from build123d import *

# Parameters (mm, degrees)
BOSS_EXTRUDE3_DEPTH              = 14.5
SKETCH8_R                        = 7.935
CUT_EXTRUDE3_DEPTH               = 88
CUT_EXTRUDE9_DEPTH               = 2.4
F_39_0_13779528_DIAMETER_HOLE1_D = 3.500000112
CUT_EXTRUDE10_DEPTH              = 22.4
CUT_EXTRUDE11_DEPTH              = 2.4
BOSS_EXTRUDE7_DEPTH              = 3.625
F_39_0_13779528_DIAMETER_HOLE2_D = 3.500000112
BOSS_EXTRUDE10_DEPTH             = 3
BOSS_EXTRUDE11_DEPTH             = 3


with BuildPart() as part:
    # Sketch6 → Boss-Extrude3 (new body)
    with BuildSketch(Plane(origin=(0, 0, 0), x_dir=(1, 0, 0), z_dir=(0, 1, 0))):
        Polygon((-16.836914056, 5.783353512), (13.163085944, 5.783353512), (20.663085944, -47.581919406), (-24.336914056, -47.581919406), align=None)
    extrude(amount=BOSS_EXTRUDE3_DEPTH)

    # Sketch8 → Cut-Extrude3 (cut)
    with BuildSketch(Plane.XY.offset(47.581919406)):
        with Locations((-1.836914056, 0)):
            Circle(SKETCH8_R)
    extrude(amount=-CUT_EXTRUDE3_DEPTH, mode=Mode.SUBTRACT)

    # Sketch18 → Cut-Extrude9 (cut)
    with BuildSketch(Plane(origin=(0, 14.5, 0), x_dir=(1, 0, 0), z_dir=(0, 1, 0))):
        Polygon((-15.771819769, -44.868285994), (-12.821819769, -43.1651027), (-12.821819769, -39.758736112), (-15.771819769, -38.055552818), (-18.721819769, -39.758736112), (-18.721819769, -43.1651027), align=None)
        Polygon((12.097991657, -44.868285994), (15.047991657, -43.1651027), (15.047991657, -39.758736112), (12.097991657, -38.055552818), (9.147991657, -39.758736112), (9.147991657, -43.1651027), align=None)
        Polygon((11.389331688, -26.016021021), (14.389331688, -24.283970214), (14.389331688, -20.819868599), (11.389331688, -19.087817791), (8.389331688, -20.819868599), (8.389331688, -24.283970214), align=None)
        Polygon((-15.0631598, -26.016021021), (-12.0631598, -24.283970214), (-12.0631598, -20.819868599), (-15.0631598, -19.087817791), (-18.0631598, -20.819868599), (-18.0631598, -24.283970214), align=None)
    extrude(amount=-CUT_EXTRUDE9_DEPTH, mode=Mode.SUBTRACT)

    # #39 (0.13779528) Diameter Hole1 (through all)
    with Locations(Plane(origin=(-15.0631598, 14.5, 22.551919406), x_dir=(0, 0, 1), z_dir=(0, 1, 0))):
        with Locations((0, 0), (0, 26.452491488), (18.91, -0.708659969), (18.91, 27.161151457)):
            Hole(F_39_0_13779528_DIAMETER_HOLE1_D / 2)

    # Sketch22 → Cut-Extrude10 (cut)
    with BuildSketch(Plane(origin=(0, 14.5, 0), x_dir=(1, 0, 0), z_dir=(0, 1, 0))):
        Polygon((-22.781301734, -36.51316259), (19.107473622, -36.51316259), (13.163085944, 5.783353512), (-16.836914056, 5.783353512), align=None)
    extrude(amount=-CUT_EXTRUDE10_DEPTH, mode=Mode.SUBTRACT)

    # Sketch24 → Cut-Extrude11 (cut)
    with BuildSketch(Plane.XZ):
        Polygon((-15.771819769, 38.055552818), (-12.821819769, 39.758736112), (-12.821819769, 43.1651027), (-15.771819769, 44.868285994), (-18.721819769, 43.1651027), (-18.721819769, 39.758736112), align=None)
        Polygon((12.097991657, 38.055552818), (15.047991657, 39.758736112), (15.047991657, 43.1651027), (12.097991657, 44.868285994), (9.147991657, 43.1651027), (9.147991657, 39.758736112), align=None)
    extrude(amount=-CUT_EXTRUDE11_DEPTH, mode=Mode.SUBTRACT)

    # Sketch27 → Boss-Extrude7 (add)
    with BuildSketch(Plane(origin=(0, 0, 0), x_dir=(1, 0, 0), z_dir=(0, 1, 0))):
        Polygon((6.098085944, -47.581919406), (20.663085944, -47.581919406), (20.663085944, -112.581919406), (-9.771914056, -112.581919406), (-24.336914056, -112.581919406), (-24.336914056, -47.581919406), (-9.771914056, -47.581919406), (-9.771914056, -97.661919406), (6.098085944, -97.661919406), align=None)
    extrude(amount=BOSS_EXTRUDE7_DEPTH)

    # #39 (0.13779528) Diameter Hole2 (through all)
    with Locations(Plane(origin=(-16.086914056, 3.625, 80.900195398), x_dir=(0, 0, 1), z_dir=(0, 1, 0))):
        with Locations((0, 0), (24.681724008, 14.25), (0, 28.5)):
            Hole(F_39_0_13779528_DIAMETER_HOLE2_D / 2)

    # Sketch39 → Boss-Extrude10 (add)
    with BuildSketch(Plane(origin=(20.663085944, 0, 0), x_dir=(0, 0, -1), z_dir=(1, 0, 0))):
        Polygon((-47.581919406, 14.5), (-112.581919406, 3.625), (-47.581919406, 3.625), align=None)
    extrude(amount=-BOSS_EXTRUDE10_DEPTH)

    # Sketch40 → Boss-Extrude11 (add)
    with BuildSketch(Plane.ZY.offset(24.336914056)):
        Polygon((47.581919406, 14.5), (112.581919406, 3.625), (47.581919406, 3.625), align=None)
    extrude(amount=-BOSS_EXTRUDE11_DEPTH)


solid = part.part
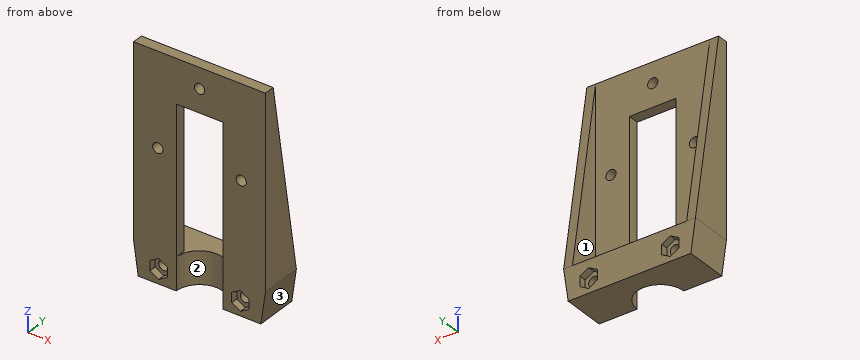
Part model, mm, in its own coordinate system. Face numbers are marked on the shaded views. A direction names the side the tool comes from. Round coordinates to 2 decimals unless told otherwise and drop trailing zeros. Loops run counter-clockwise (first coordinate to the right, second up) from the corner with the lowest first, then second, coordinate; pieces in that order, holes last. Notation, with made-up numbers: (84, -10) - (105, -10) arc R15 ccw to (105, -5) - close; hole circle Ø5 at (-9, 87). An arc over 180 degrees is marked (long way). Answer as a JSON object with one key per item and string values.
Item 1: Tool access for the marked faces 1, 2 and 3: list every direction of +Z, -Z, +X, -X, +Y, -Y with a clear straight run to the whole face (end or side of a thin tool).
Output:
{"face 1": "+Z, +Y", "face 2": "-Z, -Y", "face 3": "-Z, +X, +Y, -Y"}
Item 2: Wall check: L1, parallel to X at y = 4, z = 94; L2, parallel to X at y = 1, z = 73.5; L3, parallel to Y at x = 8.5, z = 105 (3 decimals). Give the ranges that are in metal, low to high.
Output:
{"L1": "-24.34 to -21.34, 17.66 to 20.66", "L2": "-24.34 to -9.77, 6.1 to 20.66", "L3": "0 to 3.625"}
Item 3: Band-saw the part on C-C on x = -4.5. List the corners of the cut face in (y, z) (3 decimals), plus the area to 3 significant figures.
Output:
{"outline": "(0, 97.662) - (3.625, 97.662) - (3.625, 112.582) - (0, 112.582) - close; (7.475, 36.513) - (14.5, 36.513) - (14.5, 47.582) - (7.475, 47.582) - close", "area": "132 mm2"}
Item 4: Band-saw the part on B-B on z = 88. List the corners of the cut face in (x, y) (3 decimals), plus the area to 3 significant figures.
Output:
{"outline": "(-24.337, 0) - (-9.772, 0) - (-9.772, 3.625) - (-21.337, 3.625) - (-21.337, 7.738) - (-24.337, 7.738) - close; (6.098, 0) - (20.663, 0) - (20.663, 7.738) - (17.663, 7.738) - (17.663, 3.625) - (6.098, 3.625) - close", "area": "130 mm2"}
Item 5: Band-saw the part on D-D on y = 9.75. List the corners of the cut face in (x, z), plus the area to 3 significant figures.
Output:
{"outline": "(-24.34, 47.58) - (-22.78, 36.51) - (19.11, 36.51) - (20.66, 47.58) - (20.66, 75.97) - (17.66, 75.97) - (17.66, 47.58) - (-21.34, 47.58) - (-21.34, 75.97) - (-24.34, 75.97) - close; hole circle Ø3.5 at (-15.77, 41.46); hole circle Ø3.5 at (12.1, 41.46)", "area": "632 mm2"}
Item 6: Band-saw the part on A-A on y = 6.25. List the corners of the cut face in (x, z).
Output:
{"outline": "(-24.34, 47.58) - (-22.78, 36.51) - (-6.73, 36.51) - (-6.73, 47.58) - (-21.34, 47.58) - (-21.34, 96.89) - (-24.34, 96.89) - close; (3.05, 36.51) - (19.11, 36.51) - (20.66, 47.58) - (20.66, 96.89) - (17.66, 96.89) - (17.66, 47.58) - (3.05, 47.58) - close; hole circle Ø3.5 at (-15.77, 41.46); hole circle Ø3.5 at (12.1, 41.46)"}
Item 7: Pin check, flat tips, straight feed: pin 1 (11.5 mm diameter, centred on x = 4.5, z = 80, fed in from +Y) (3 decimals); pin 2 (3 mm diameter, centred on x = 12, z = 42, fed in from -Y); pin 3 (3 mm diameter, centred on x = 12.1, z = 41.46, fed in from +Y); pin 4 (1.2 mm diameter, centred on y = 1, z = 41.5, fed in from -X). Stop position of each tip, or through.
Output:
{"pin 1": "y = 3.625", "pin 2": "y = 2.4", "pin 3": "through", "pin 4": "x = -23.57"}
